from build123d import *

# Parameters (mm, degrees)
SKETCH1_W           = 72
SKETCH1_H           = 82
BOSS_EXTRUDE1_DEPTH = 2
BOSS_EXTRUDE2_START = -2
SKETCH2_W           = 78
SKETCH2_H           = 88
BOSS_EXTRUDE2_DEPTH = 64
SKETCH4_R           = 8.5
CUT_EXTRUDE1_DEPTH  = 3


with BuildPart() as part:
    # Sketch1 → Boss-Extrude1 (new body)
    with BuildSketch(Plane(origin=(0, 0, 0), x_dir=(1, 0, 0), z_dir=(0, 1, 0))):
        with Locations((36, 41)):
            Rectangle(SKETCH1_W, SKETCH1_H)
    extrude(amount=BOSS_EXTRUDE1_DEPTH)

    # Sketch2 → Boss-Extrude2 (add)
    with BuildSketch(Plane(origin=(0, 2, 0), x_dir=(1, 0, 0), z_dir=(0, 1, 0)).offset(BOSS_EXTRUDE2_START)):
        with Locations((36, 41)):
            Rectangle(SKETCH2_W, SKETCH2_H)
        Polygon((5, 82), (67, 82), (67, 77), (72, 77), (72, 5), (67, 5), (67, 0), (5, 0), (5, 5), (0, 5), (0, 77), (5, 77), align=None, mode=Mode.SUBTRACT)
    extrude(amount=BOSS_EXTRUDE2_DEPTH)

    # Sketch4 → Cut-Extrude1 (cut)
    with BuildSketch(Plane.XY.offset(3)):
        with Locations((36, 64)):
            Circle(SKETCH4_R)
    extrude(amount=-CUT_EXTRUDE1_DEPTH, mode=Mode.SUBTRACT)


solid = part.part
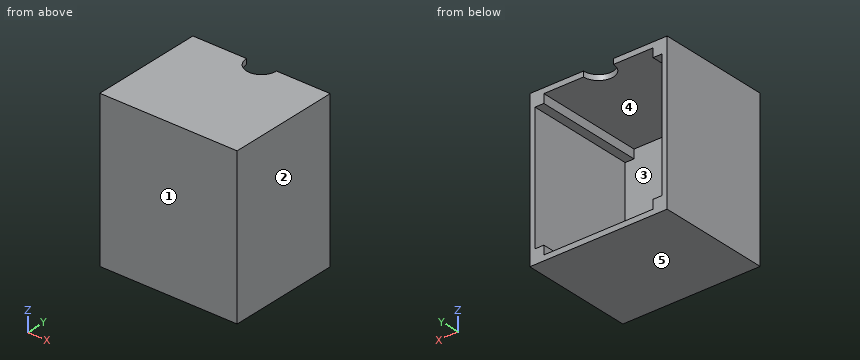
The model under review builds one solid part; all positions refer to its coordinate system, in mm. Face numbers are marked on the shaded views. A direction names the side the tool comes from. Give positions to 0.01 mm unless a question says otherwise; leave off trailing zeros. Order: outer loops, then holes, each group sorted by start corner. A loop starts at its lowest first (then second) coordinate and runs counter-clockwise, first axis right, second up. Notation, with made-up numbers: M -27,-32 L -19,-32 A25 cw -19,-9 Z; hole C -4.75,53.5 d4. An arc over 180 degrees is marked long. Answer in a Markdown table with one row per item. Add a question column.
1. Add section C-C on y = 53.5. State the section outline as (x, z) points.
2. Mouldability with a two-part tool opening along X and no side actions: class the marked faces 1, 2 and 3 as released by +X, released by -X, zero draft, split by the parting line, or undercut.
3. To check wall thickness, follow line 1 along X through (y, z) = (21.5, -59); line 2 along Z through (x, y) = (9.5, 37); line 3 along Z through (x, y) = (70.5, 9). State the ranges of each line that lie inside material, in increasing order.
4. Add section B-B on x = 47. State the section outline as (y, z) points, plus the area to 3 significant figures.
5. For pin 1 Ø6 at (x, z) = (25.5, -68) entering from +Y, flat-tipped, find the tip position at first contact; note if it passes through.
6. Add section A-A on z = -39. State the section outline as (x, y) points.
7. Machinability: for the marked faces 4 and 5, which of the approach directions +Z, -Z, +X, -X, +Y, -Y give a long, thin tool a straight path to every point of the face, cutting with its end or side? Answer none if there is none.
The answers:
| question | item | result |
|---|---|---|
| 1 | outline | M -3,-85 L 75,-85 L 75,3 L -3,3 Z; hole M 0,-77 L 5,-77 L 5,-82 L 67,-82 L 67,-77 L 72,-77 L 72,-5 L 67,-5 L 67,0 L 5,0 L 5,-5 L 0,-5 Z |
| 2 | face 1 | zero draft |
| 2 | face 2 | released by +X |
| 2 | face 3 | undercut |
| 3 | line 1 | -3 to 0, 72 to 75 |
| 3 | line 2 | -85 to -82, 0 to 3 |
| 3 | line 3 | -85 to -77, -5 to 3 |
| 4 | outline | M 0,-85 L 64,-85 L 64,-82 L 2,-82 L 2,0 L 64,0 L 64,3 L 0,3 Z |
| 4 | area | 548 mm2 |
| 5 | pin 1 | y = 2 |
| 6 | outline | M -3,0 L 75,0 L 75,64 L 72,64 L 72,2 L 0,2 L 0,64 L -3,64 Z |
| 7 | face 4 | +Y |
| 7 | face 5 | -Z, +X, -X, +Y, -Y |
